from build123d import *

# Parameters (mm, degrees)
SKETCH1_R                      = 4
BOSS_EXTRUDE1_DEPTH            = 3
BOSS_EXTRUDE3_DEPTH            = 20
BOSS_EXTRUDE4_START            = 30
SKETCH4_W                      = 36.05
SKETCH4_H                      = 4
BOSS_EXTRUDE4_DEPTH            = 30
SKETCH6_W                      = 36.05
SKETCH6_H                      = 4
BOSS_EXTRUDE5_DEPTH            = 16
CUT_EXTRUDE2_REACH             = 109.19
SKETCH5_R                      = 2.5
SKETCH5_R_2                    = 3
CUT_EXTRUDE2_DIRECTION_2_REACH = 109.19


with BuildPart() as part:
    # Sketch1 → Boss-Extrude1 (new body)
    with BuildSketch(Plane(origin=(0, 0, 0), x_dir=(1, 0, 0), z_dir=(0, 1, 0))):
        with BuildLine():
            Line((-18.025, 0), (-18.025, 97.29))
            ThreePointArc((-18.025, 97.29), (0, 115.315), (18.025, 97.29))
            Line((18.025, 97.29), (18.025, 0))
            ThreePointArc((18.025, 0), (0, -18.025), (-18.025, 0))
        make_face()
        with Locations(Location((0, 0, 0), (0, 0, 270))):
            Circle(SKETCH1_R, mode=Mode.SUBTRACT)
        with Locations(Location((0, 97.29, 0), (0, 0, 90))):
            Circle(SKETCH1_R, mode=Mode.SUBTRACT)
    boss_extrude1 = extrude(amount=BOSS_EXTRUDE1_DEPTH)

    # Sketch3 → Boss-Extrude3 (add)
    with BuildSketch(Plane(origin=(0, 3, 0), x_dir=(1, 0, 0), z_dir=(0, 1, 0))):
        with BuildLine():
            Line((-15.025, 0), (-18.025, 0))
            ThreePointArc((-18.025, 0), (0, -18.025), (18.025, 0))
            Line((18.025, 0), (18.025, 97.29))
            ThreePointArc((18.025, 97.29), (12.745599731, 110.035599731), (0, 115.315))
            Line((0, 115.315), (0, 112.315))
            ThreePointArc((0, 112.315), (10.624279387, 107.914279387), (15.025, 97.29))
            Line((15.025, 97.29), (15.025, 0))
            ThreePointArc((15.025, 0), (0, -15.025), (-15.025, 0))
        make_face()
    extrude(amount=BOSS_EXTRUDE3_DEPTH)

    # Mirror1: Boss-Extrude1 across plane
    add(boss_extrude1.mirror(Plane.ZX.offset(13)))

    # Sketch4 → Boss-Extrude4 (add)
    with BuildSketch(Plane.XZ.offset(BOSS_EXTRUDE4_START)):
        with Locations((0, -12)):
            Rectangle(SKETCH4_W, SKETCH4_H)
        with BuildLine():
            Line((-14.996687134, 10), (14.996687134, 10))
            ThreePointArc((14.996687134, 10), (13.326001448, 12.137475454), (11.353441108, 14))
            Line((11.353441108, 14), (-11.353441108, 14))
            ThreePointArc((-11.353441108, 14), (-13.326001448, 12.137475454), (-14.996687134, 10))
        make_face()
    boss_extrude4 = extrude(amount=-BOSS_EXTRUDE4_DEPTH)

    # Sketch6 → Boss-Extrude5 (add)
    with BuildSketch(Plane.XZ):
        with Locations((0, -12)):
            Rectangle(SKETCH6_W, SKETCH6_H)
        with Locations((0, -85.29)):
            Rectangle(SKETCH6_W, SKETCH6_H)
    boss_extrude5 = extrude(amount=BOSS_EXTRUDE5_DEPTH)

    # Cut-Extrude2: up to this face of the body (flat: up to its plane)
    cut_extrude2_end = Plane(part.part.faces().sort_by_distance((0, -15, 14))[0])
    # Sketch5 → Cut-Extrude2 (cut, up to the picked face)
    with BuildSketch(Plane(origin=(0, 0, -14), x_dir=(-1, 0, 0), z_dir=(0, 0, -1)), mode=Mode.PRIVATE) as cut_extrude2_sk1:
        with Locations((0, -8)):
            Circle(SKETCH5_R)
    cut_extrude2_tool1 = split(extrude(cut_extrude2_sk1.sketch, amount=-CUT_EXTRUDE2_REACH, mode=Mode.PRIVATE), bisect_by=cut_extrude2_end, keep=Keep.BOTH, mode=Mode.PRIVATE)
    # Sketch5 → Cut-Extrude2 (cut, up to the picked face)
    with BuildSketch(Plane(origin=(0, 0, -14), x_dir=(-1, 0, 0), z_dir=(0, 0, -1)), mode=Mode.PRIVATE) as cut_extrude2_sk2:
        with Locations(Location((-9.0125, -22.5, 0), (0, 0, 218.710740726))):
            Circle(SKETCH5_R_2)
    cut_extrude2_tool2 = split(extrude(cut_extrude2_sk2.sketch, amount=-CUT_EXTRUDE2_REACH, mode=Mode.PRIVATE), bisect_by=cut_extrude2_end, keep=Keep.BOTH, mode=Mode.PRIVATE)
    # Sketch5 → Cut-Extrude2 (cut, up to the picked face)
    with BuildSketch(Plane(origin=(0, 0, -14), x_dir=(-1, 0, 0), z_dir=(0, 0, -1)), mode=Mode.PRIVATE) as cut_extrude2_sk3:
        with Locations(Location((9.0125, -22.5, 0), (0, 0, 321.289306711))):
            Circle(SKETCH5_R_2)
    cut_extrude2_tool3 = split(extrude(cut_extrude2_sk3.sketch, amount=-CUT_EXTRUDE2_REACH, mode=Mode.PRIVATE), bisect_by=cut_extrude2_end, keep=Keep.BOTH, mode=Mode.PRIVATE)
    cut_extrude2_1 = cut_extrude2_tool1.solids().sort_by(Axis((0, -8, -14), (0, 0, 1)))[0]
    add(cut_extrude2_1, mode=Mode.SUBTRACT)
    cut_extrude2_2 = cut_extrude2_tool2.solids().sort_by(Axis((9.0125, -22.5, -14), (0, 0, 1)))[0]
    add(cut_extrude2_2, mode=Mode.SUBTRACT)
    cut_extrude2_3 = cut_extrude2_tool3.solids().sort_by(Axis((-9.0125, -22.5, -14), (0, 0, 1)))[0]
    add(cut_extrude2_3, mode=Mode.SUBTRACT)
    cut_extrude2 = cut_extrude2_1 + cut_extrude2_2 + cut_extrude2_3  # Cut-Extrude2 as one shape, for the pattern or mirror that repeats it

    # Cut-Extrude2 direction 2: up to this face of the body (flat: up to its plane)
    cut_extrude2_direction_2_end = Plane(part.part.faces().sort_by_distance((0, -8, -87.29))[0])
    # Sketch5 → Cut-Extrude2 direction 2 (cut, up to the picked face)
    with BuildSketch(Plane(origin=(0, 0, -14), x_dir=(-1, 0, 0), z_dir=(0, 0, -1)), mode=Mode.PRIVATE) as cut_extrude2_direction_2_sk1:
        with Locations((0, -8)):
            Circle(SKETCH5_R)
    cut_extrude2_direction_2_tool1 = split(extrude(cut_extrude2_direction_2_sk1.sketch, amount=CUT_EXTRUDE2_DIRECTION_2_REACH, mode=Mode.PRIVATE), bisect_by=cut_extrude2_direction_2_end, keep=Keep.BOTH, mode=Mode.PRIVATE)
    # Sketch5 → Cut-Extrude2 direction 2 (cut, up to the picked face)
    with BuildSketch(Plane(origin=(0, 0, -14), x_dir=(-1, 0, 0), z_dir=(0, 0, -1)), mode=Mode.PRIVATE) as cut_extrude2_direction_2_sk2:
        with Locations(Location((-9.0125, -22.5, 0), (0, 0, 218.710740726))):
            Circle(SKETCH5_R_2)
    cut_extrude2_direction_2_tool2 = split(extrude(cut_extrude2_direction_2_sk2.sketch, amount=CUT_EXTRUDE2_DIRECTION_2_REACH, mode=Mode.PRIVATE), bisect_by=cut_extrude2_direction_2_end, keep=Keep.BOTH, mode=Mode.PRIVATE)
    # Sketch5 → Cut-Extrude2 direction 2 (cut, up to the picked face)
    with BuildSketch(Plane(origin=(0, 0, -14), x_dir=(-1, 0, 0), z_dir=(0, 0, -1)), mode=Mode.PRIVATE) as cut_extrude2_direction_2_sk3:
        with Locations(Location((9.0125, -22.5, 0), (0, 0, 321.289306711))):
            Circle(SKETCH5_R_2)
    cut_extrude2_direction_2_tool3 = split(extrude(cut_extrude2_direction_2_sk3.sketch, amount=CUT_EXTRUDE2_DIRECTION_2_REACH, mode=Mode.PRIVATE), bisect_by=cut_extrude2_direction_2_end, keep=Keep.BOTH, mode=Mode.PRIVATE)
    cut_extrude2_direction_2_1 = cut_extrude2_direction_2_tool1.solids().sort_by(Axis((0, -8, -14), (0, 0, -1)))[0]
    add(cut_extrude2_direction_2_1, mode=Mode.SUBTRACT)
    cut_extrude2_direction_2_2 = cut_extrude2_direction_2_tool2.solids().sort_by(Axis((9.0125, -22.5, -14), (0, 0, -1)))[0]
    add(cut_extrude2_direction_2_2, mode=Mode.SUBTRACT)
    cut_extrude2_direction_2_3 = cut_extrude2_direction_2_tool3.solids().sort_by(Axis((-9.0125, -22.5, -14), (0, 0, -1)))[0]
    add(cut_extrude2_direction_2_3, mode=Mode.SUBTRACT)
    cut_extrude2_direction_2 = cut_extrude2_direction_2_1 + cut_extrude2_direction_2_2 + cut_extrude2_direction_2_3  # Cut-Extrude2 direction 2 as one shape, for the pattern or mirror that repeats it

    # Mirror3: Boss-Extrude4, Boss-Extrude5, Cut-Extrude2, Cut-Extrude2 direction 2 across plane
    add(boss_extrude4.mirror(Plane.ZX.offset(13)))
    add(boss_extrude5.mirror(Plane.ZX.offset(13)))
    add(cut_extrude2.mirror(Plane.ZX.offset(13)), mode=Mode.SUBTRACT)
    add(cut_extrude2_direction_2.mirror(Plane.ZX.offset(13)), mode=Mode.SUBTRACT)


solid = part.part
Geometry check sheet. Reference: the model listing, model coordinates, mm. A direction names the side the tool comes from. Coordinates: 2 decimals unless noted, no trailing zeros. Write each loop counter-clockwise with the first axis right and the second up, starting at its lowest first coordinate (ties: lowest second). Pieces come first, ordered by that corner, then holes. Notation, with made-up numbers: (-38, 68.25) -> (2, 68.25) arc R22 cw to (2, 92.25) -> close; hole circle Ø10 at (74.5, -9). An arc over 180 degrees is marked (long way). One line per question, with ' | ' between items.
1. Cross-section at A-A on y = 34. Record the cut outline in (x, z) (3 decimals).
Answers:
outline: (-18.025, -87.29) -> (-2.5, -87.29) -> (-2.5, -83.29) -> (-18.025, -83.29) -> close; (-18.025, -14) -> (-2.5, -14) -> (-2.5, -10) -> (-18.025, -10) -> close; (-14.997, 10) -> (-2.5, 10) -> (-2.5, 14) -> (-11.353, 14) arc R18.025 ccw to start; (2.5, -87.29) -> (18.025, -87.29) -> (18.025, -83.29) -> (2.5, -83.29) -> close; (2.5, -14) -> (18.025, -14) -> (18.025, -10) -> (2.5, -10) -> close; (2.5, 10) -> (14.997, 10) arc R18.025 ccw to (11.353, 14) -> (2.5, 14) -> close
2. Cross-section at B-B on z = -95. Record the cut outline in (x, y) (3 decimals), and give its area (3 significant figures).
Answers:
outline: (-18.025, 0) -> (-3.28, 0) -> (-3.28, 3) -> (-18.025, 3) -> close; (-18.025, 23) -> (-3.28, 23) -> (-3.28, 26) -> (-18.025, 26) -> close; (3.28, 0) -> (18.025, 0) -> (18.025, 26) -> (3.28, 26) -> (3.28, 23) -> (15.025, 23) -> (15.025, 3) -> (3.28, 3) -> close | area: 237 mm²
3. Draft check along X on faces 1 (the flat face through (-18.025, 1, -45)), 2 (the flat face through (0, -16, -85)), 3 (the cylindrical face through (0.33, 31.52, -12.03)), 4 (the cylindrical face through (8.689, 51.483, -12.028)). Enter one of: +X half, -X half, draft (parallel to the pull), parting line (faces both ways), or undercut.
Answers:
face 1: -X half | face 2: draft | face 3: undercut | face 4: undercut
4. Thickness scan on probe 1 along X at (y, z) = (-22.5, -11.7) (1 decimal); probe 2 along Z at (x, y) = (-5, 27.5); probe 3 along Y at (x, z) = (0, -12.3). Record the ranges inside material, lowest first. Write a range as from..to.
Answers:
probe 1: x = -18..-12, -6..6, 12..18 | probe 2: z = -87.29..-83.29, -14..-10, 10..14 | probe 3: y = -30..-10.5, -5.5..3, 23..31.5, 36.5..56
5. Set-up check for faces 5 (the flat face through (0, 41, -10)), 6 (the cylindrical face through (0.33, 12.86, 15.02)), 7 (the flat face through (0, 13, -114)), 8 (the flat face through (0, -15, -10)), 9 (the flat face through (0, -4, -87.29)): record each of +Z, -Z, +X, -X, +Y, -Y from which the full face is reachable in a straight line by a thin tool's end or side.
Answers:
face 5: +X, -X, +Y | face 6: none | face 7: -Z, -X | face 8: +X, -X, -Y | face 9: -Z, +X, -X, -Y
6. Cross-section at D-D on x = 9. State how many separate pieces and enclosed holes the cut face has, and give its area (3 significant figures).
Answers:
separate pieces: 5 | enclosed holes: 1 | area: 1,430 mm²
7. Depth check by flat-ended pin: pin 1 Ø4 at (x, y) = (1, 35.5) entering from +Z; pin 2 Ø5 at (x, y) = (-5.5, -11) entering from -Z; pin 3 Ø4.5 at (x, y) = (0, -8) entering from -Z; pin 4 Ø2.5 at (x, y) = (-16.5, 13) entering from -Z. Enter the tip coordinate at first touch or a pass-through.
Answers:
pin 1: stops at z = 14 | pin 2: stops at z = -87.29 | pin 3: passes through | pin 4: stops at z = 0
8. Cross-section at C-C on z = -73.5. Record the cut outline in (x, y) (3 decimals), and give its area (3 significant figures).
Answers:
outline: (-18.025, 0) -> (18.025, 0) -> (18.025, 26) -> (-18.025, 26) -> (-18.025, 23) -> (15.025, 23) -> (15.025, 3) -> (-18.025, 3) -> close | area: 276 mm²
